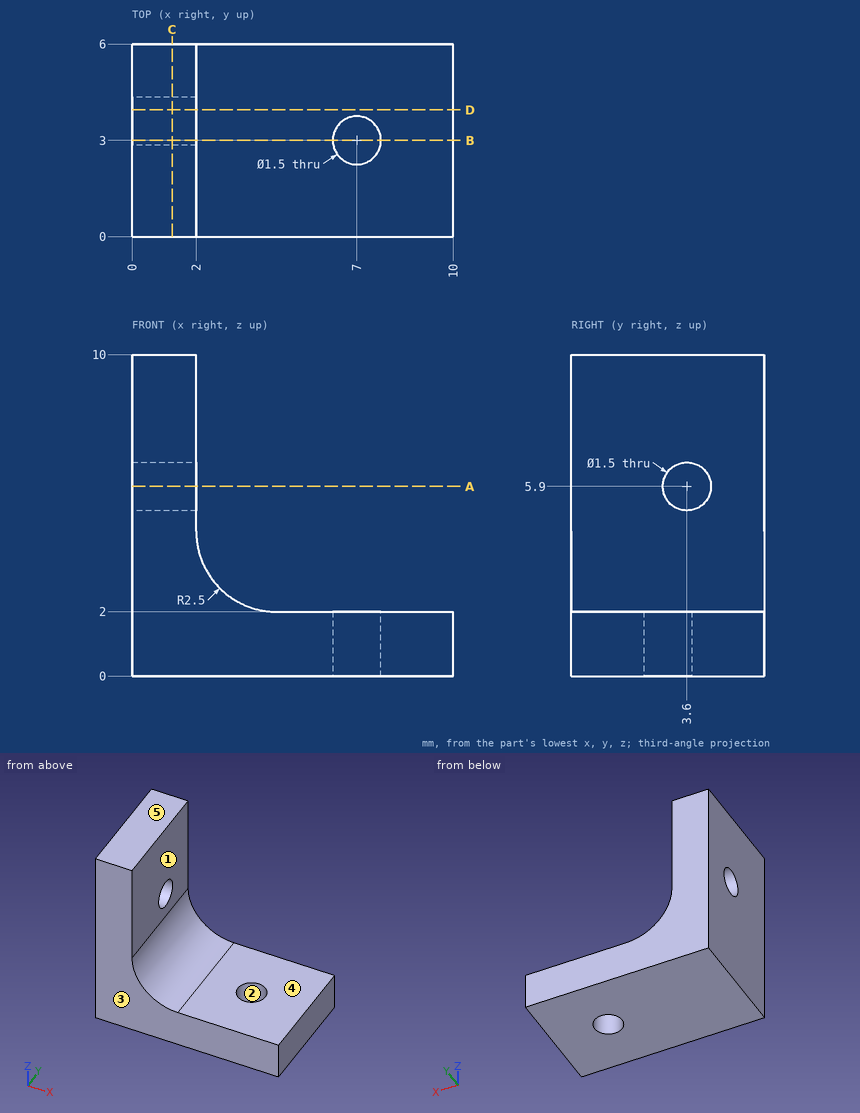
Could you check a few things on this drawing? It's one solid part, dimensions in mm from its lowest x, y, z. A direction names the side the tool comes from. Coordinates: 2 decimals unless noted, no trailing zeros. Order: outer loops, then holes, each group sorted by start corner. A loop starts at its lowest first (then second) coordinate and runs counter-clockwise, first axis right, second up. Notation, with made-up numbers: (29, -7.5) - (72, -7.5) arc R27 ccw to (72, 15.5) - close; hole circle Ø3 at (52.25, 16). An arc over 180 degrees is marked (long way). One line per question, with ' | ' between items. Start each with the question number.
1. If we section it at A-A (z = 5.9): Write out the boundary of the cut face in (x, y).
2. If we section it at B-B (y = 3): Write out the boundary of the cut face in (x, z), and give its area (3 significant figures).
3. If we section it at D-D (y = 3.95): Write out the boundary of the cut face in (x, z), and give its area (3 significant figures).
4. If we mould it in two halves opening along X, with no side actions, what happens to the marked faces 1, 2 and 3? For each: released by +X, released by -X, zero draft, split by the parting line, or undercut.
5. If we section it at C-C (x = 1.25): Write out the boundary of the cut face in (y, z).
6. I'm going to push flat-ended pins straight in: pin 1 Ø2 at (x, y) = (7, 3) entering from -Z; pin 2 Ø1.6 at (x, y) = (6.5, 4) entering from +Z. Where does each tip first touch, or does it pass through?
7. Please list where these lines run through material, in increasing order: line 1 along Y through (x, z) = (1.2, 5.9); line 2 along Y through (x, z) = (7, 0.4); line 3 along X through (y, z) = (1.2, 6.75). Write a range as [from, to].
8. Which directions (+Z, -Z, +X, -X, +Y, -Y) give clear straight access to the entire face, cutting with the end or side of a thin tool? Please do the marked faces 4 and 5.
Model answer:
1) outline: (0, 0) - (2, 0) - (2, 2.85) - (0, 2.85) - close; (0, 4.35) - (2, 4.35) - (2, 6) - (0, 6) - close
2) outline: (0, 0) - (6.25, 0) - (6.25, 2) - (4.5, 2) arc R2.5 cw to (2, 4.5) - (2, 5.45) - (0, 5.45) - close; (0, 6.35) - (2, 6.35) - (2, 10) - (0, 10) - close; (7.75, 0) - (10, 0) - (10, 2) - (7.75, 2) - close | area: 32.5 mm²
3) outline: (0, 0) - (10, 0) - (10, 2) - (4.5, 2) arc R2.5 cw to (2, 4.5) - (2, 5.24) - (0, 5.24) - close; (0, 6.56) - (2, 6.56) - (2, 10) - (0, 10) - close | area: 34.7 mm²
4) face 1: released by +X | face 2: undercut | face 3: zero draft
5) outline: (0, 0) - (6, 0) - (6, 10) - (0, 10) - close; hole circle Ø1.5 at (3.6, 5.9)
6) pin 1: stops at z = 0 | pin 2: stops at z = 2
7) line 1: y = [0, 2.85], [4.35, 6] | line 2: y = [0, 2.25], [3.75, 6] | line 3: x = [0, 2]
8) face 4: +Z, +X, +Y, -Y | face 5: +Z, +X, -X, +Y, -Y
